Input: dimensioned drawing with shaded views. Units: mm. Origin: part minimum x, y, z. A direction names the side the tool comes from. Round coordinates to 2 decimals unless told otherwise and drop trailing zeros. Write each loop counter-clockwise with the first axis right and the second up, starting at its lowest first coordinate (ties: lowest second). Pieces come first, ordered by that corner, then holes. Notation, with made-up numbers: M 74.5,22 L 116.5,22 A19 cw 116.5,30 Z; hole C 0,26.25 d5. An arc over 180 degrees is marked long. Answer in a Markdown table with one row per item. Add a question column.
Item 1: Mould query, pull axis Z, two halves, no side actions, for the marked faces 6, 7 and 8. Classes: released by +Z, released by -Z, zero draft, split by the parting line, or undercut.
Item 2: Contact query for flat-ended pins moving along their axis: pin 1 (2 mm diameter, centred on x = 2.5, z = 16.5, fed in from +Y); pin 2 (5 mm diameter, centred on y = 8.5, z = 11.5, fed in from -X); pin 3 (1 mm diameter, centred on x = 2, z = 7, fed in from +Y). Output: stop coordinate, or through.
Item 3: Cut plane D-D on z = 15.25. Return loops of the section in (x, y).
Item 4: Cut plane A-A on y = 4.85. Return loops of the section in (x, z).
Item 5: Cut plane C-C on z = 3.75. Return loops of the section in (x, y).
Item 6: Set-up query: the marked faces 1, 2, 3, 4 and 5. Return all of +Z, -Z, +X, -X, +Y, -Y with unobstructed straight access to the full face (end or side cutting, diameter ignored); none if empty.
Item 7: Material intervals for probe 1 along Z at (x, y) = (3, 2.5); probe 2 along Y at (x, z) = (4.75, 7.5); probe 3 along Z at (x, y) = (8.75, 5), sorted ascending.
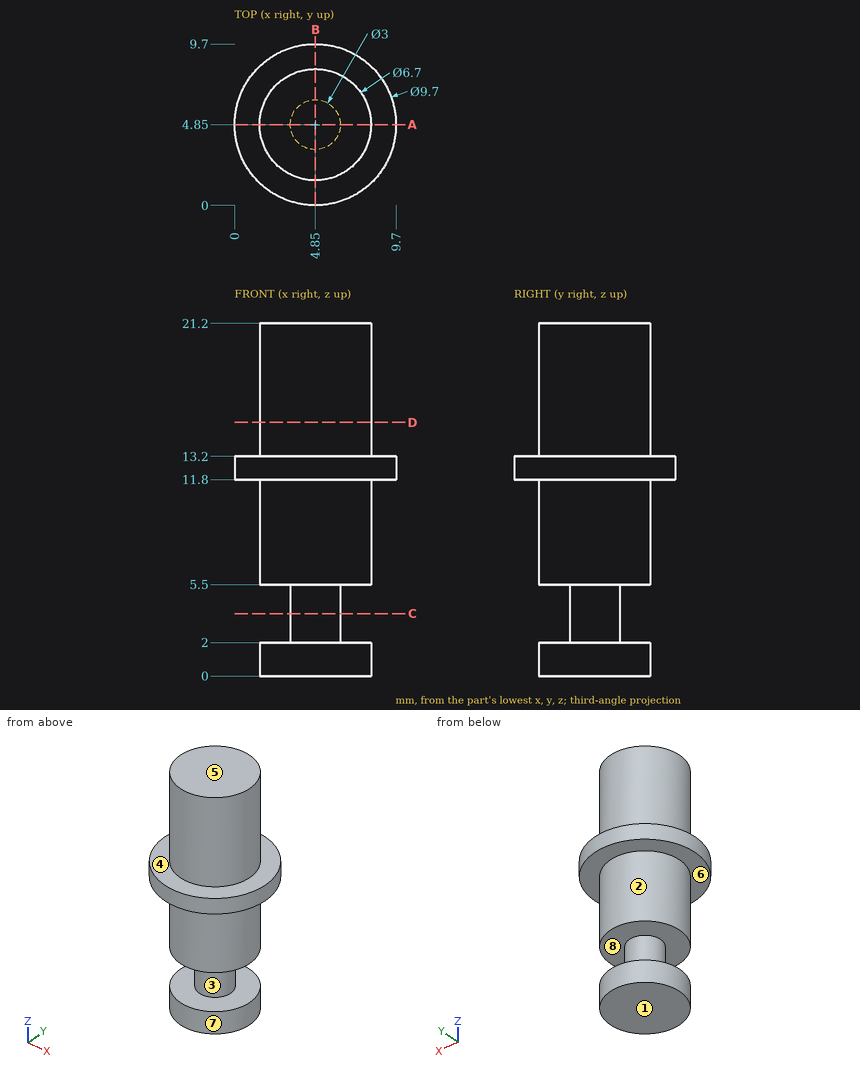
Results below:
| question | item | result |
|---|---|---|
| 1 | face 6 | released by -Z |
| 1 | face 7 | zero draft |
| 1 | face 8 | undercut |
| 2 | pin 1 | y = 7.92 |
| 2 | pin 2 | x = 0.14 |
| 2 | pin 3 | y = 7.24 |
| 3 | outline | C 4.85,4.85 d6.7 |
| 4 | outline | M 0,11.8 L 1.5,11.8 L 1.5,5.5 L 3.35,5.5 L 3.35,2 L 1.5,2 L 1.5,0 L 8.2,0 L 8.2,2 L 6.35,2 L 6.35,5.5 L 8.2,5.5 L 8.2,11.8 L 9.7,11.8 L 9.7,13.2 L 8.2,13.2 L 8.2,21.2 L 1.5,21.2 L 1.5,13.2 L 0,13.2 Z |
| 5 | outline | C 4.85,4.85 d3 |
| 6 | face 1 | -Z, +X, -X, +Y, -Y |
| 6 | face 2 | -Z |
| 6 | face 3 | none |
| 6 | face 4 | +Z |
| 6 | face 5 | +Z, +X, -X, +Y, -Y |
| 7 | probe 1 | 0 to 2, 5.5 to 21.2 |
| 7 | probe 2 | 1.5 to 8.2 |
| 7 | probe 3 | 11.8 to 13.2 |
